from build123d import *

# Parameters (mm, degrees)
EXTRUDE_THIN1_DEPTH = 44
SKETCH2_R           = 2.58
CUT_EXTRUDE1_DEPTH  = 10
FILLET1_R           = 18
FILLET2_R           = 18
FILLET3_R           = 18
FILLET4_R           = 18
FILLET5_R           = 1
FILLET6_R           = 1
SKETCH11_R          = 5
SKETCH11_R_2        = 0.6
CUT_EXTRUDE2_DEPTH  = 10
SKETCH12_R          = 5
SKETCH12_R_2        = 0.6
CUT_EXTRUDE3_DEPTH  = 10


with BuildPart() as part:
    # Sketch1 → Extrude-Thin1 (new body)
    with BuildSketch(Plane(origin=(0, 0, 0), x_dir=(1, 0, 0), z_dir=(0, 1, 0))):
        Polygon((31, 57), (31, 0), (-31, 0), (-31, 57), (-32, 57), (-32, -1), (32, -1), (32, 57), align=None)
    extrude(amount=EXTRUDE_THIN1_DEPTH)

    # Sketch2 → Cut-Extrude1 (cut)
    with BuildSketch(Plane(origin=(32, 0, 0), x_dir=(0, 0, -1), z_dir=(1, 0, 0))):
        with Locations((39, 22)):
            Circle(SKETCH2_R)
    extrude(amount=-CUT_EXTRUDE1_DEPTH, mode=Mode.SUBTRACT)

    # Fillet1
    fillet1_edges = [part.edges().sort_by_distance(p)[0] for p in [
        (31.5, 0, -57),
    ]]
    fillet(fillet1_edges, radius=FILLET1_R)

    # Fillet2
    fillet2_edges = [part.edges().sort_by_distance(p)[0] for p in [
        (31.5, 44, -57),
    ]]
    fillet(fillet2_edges, radius=FILLET2_R)

    # Fillet3
    fillet3_edges = [part.edges().sort_by_distance(p)[0] for p in [
        (-31.5, 44, -57),
    ]]
    fillet(fillet3_edges, radius=FILLET3_R)

    # Fillet4
    fillet4_edges = [part.edges().sort_by_distance(p)[0] for p in [
        (-31.5, 0, -57),
    ]]
    fillet(fillet4_edges, radius=FILLET4_R)

    # Fillet5
    fillet5_edges = [part.edges().sort_by_distance(p)[0] for p in [
        (-32, 22, 1),
    ]]
    fillet(fillet5_edges, radius=FILLET5_R)

    # Fillet6
    fillet6_edges = [part.edges().sort_by_distance(p)[0] for p in [
        (32, 22, 1),
    ]]
    fillet(fillet6_edges, radius=FILLET6_R)

    # Sketch11 → Cut-Extrude2 (cut)
    with BuildSketch(Plane.ZY.offset(32)):
        with Locations((-38.961003009, 22)):
            Circle(SKETCH11_R)
        with Locations((-38.961003009, 30)):
            Circle(SKETCH11_R_2)
        with Locations((-30.961003009, 22)):
            Circle(SKETCH11_R_2)
        with Locations((-38.961003009, 14)):
            Circle(SKETCH11_R_2)
        with Locations((-46.961003009, 22)):
            Circle(SKETCH11_R_2)
        with Locations((-44.617857259, 27.656854249)):
            Circle(SKETCH11_R_2)
        with Locations((-33.30414876, 27.656854249)):
            Circle(SKETCH11_R_2)
        with Locations((-33.30414876, 16.343145751)):
            Circle(SKETCH11_R_2)
        with Locations((-44.617857259, 16.343145751)):
            Circle(SKETCH11_R_2)
    extrude(amount=-CUT_EXTRUDE2_DEPTH, mode=Mode.SUBTRACT)

    # Sketch12 → Cut-Extrude3 (cut)
    with BuildSketch(Plane.XY.offset(1)):
        with Locations((0, 22)):
            Circle(SKETCH12_R)
        with Locations((0, 30)):
            Circle(SKETCH12_R_2)
        with Locations((5.656854249, 27.656854249)):
            Circle(SKETCH12_R_2)
        with Locations((8, 22)):
            Circle(SKETCH12_R_2)
        with Locations((5.656854249, 16.343145751)):
            Circle(SKETCH12_R_2)
        with Locations((0, 14)):
            Circle(SKETCH12_R_2)
        with Locations((-5.656854249, 16.343145751)):
            Circle(SKETCH12_R_2)
        with Locations((-8, 22)):
            Circle(SKETCH12_R_2)
        with Locations((-5.656854249, 27.656854249)):
            Circle(SKETCH12_R_2)
    extrude(amount=-CUT_EXTRUDE3_DEPTH, mode=Mode.SUBTRACT)


solid = part.part
Build history of the part. All positions in model axes, mm. A direction names the side the tool comes from. Round coordinates to 2 decimals unless told otherwise and drop trailing zeros. Write each loop counter-clockwise with the first axis right and the second up, starting at its lowest first coordinate (ties: lowest second). Pieces come first, ordered by that corner, then holes. Notation, with made-up numbers: M 33.25,-5 L 56.25,-5 A7 cw 56.25,5 Z; hole C -9.75,-7 d2. An arc over 180 degrees is marked long. Answer as a JSON object with one key per item and string values. Group by question number.
(1) Cut at C-C (y = 41). Give the cut face in (x, z), and give its area (3 significant figures).
(2) Flat gauge pins, fed straight in: pin 1 (16 mm diameter, centred on x = 0, y = 22, fed in from -Z); pin 2 (0.7 mm diameter, centred on y = 22, z = -30.96, fed in from -X). Where does each tip first touch, or does it go through?
(3) Cut at D-D (x = -21). Give the cut face in (y, z).
(4) Cut at B-B (x = -2.5). Give the cut face in (y, z), and give its area (3 significant figures).
(5) Mould opens along X. For faces 1 (the flat face through (32, 22, -28)), 2 (the cylindrical face through (-1.08, 17.12, 0.51)), 3 (the cylindrical face through (-31.507, 17.564, -36.654)) say: pulls with the +X half, pulls with the -X half, needs draft (parallel to the pull), parting line crosses it, or undercut.
(6) Which spindle directions (+Z, -Z, +X, -X, +Y, -Y) get a long thin tool onto all of the face, cutting with end or side? Do faces 4 (the flat face through (31, 22, -29)), 5 (the flat face through (-0.4, 16.8, 1)). Say none if no direction does.
(7) Drill centre lines: L1, parallel to X at y = 35.5, z = -34.5; L2, parallel to Z at x = 19.5, y = 3.5. Where is each one in solid material? Low to high.
(8) Cut at A-A (z = -7). Give the cut face in (x, y), and give its area (3 significant figures).
Responses:
{
 "1": {"outline": "M -32,-48.95 L -31,-48.95 L -31,0 L 31,0 L 31,-48.95 L 32,-48.95 L 32,0 A1 ccw 31,1 L -31,1 A1 ccw -32,0 Z", "area": "161 mm2"},
 "2": {"pin 1": "stops at z = 0", "pin 2": "stops at x = 31"},
 "3": {"outline": "M 0,0 L 44,0 L 44,1 L 0,1 Z"},
 "4": {"outline": "M 0,0 L 17.67,0 L 17.67,1 L 0,1 Z; M 26.33,0 L 44,0 L 44,1 L 26.33,1 Z", "area": "35.3 mm2"},
 "5": {"face 1": "pulls with the +X half", "face 2": "undercut", "face 3": "needs draft"},
 "6": {"face 4": "-Z, +Y, -Y", "face 5": "+Z, +X, -X, +Y, -Y"},
 "7": {"L1": "x = -32 to -31, 31 to 32", "L2": "z = 0 to 1"},
 "8": {"outline": "M -32,0 L -31,0 L -31,44 L -32,44 Z; M 31,0 L 32,0 L 32,44 L 31,44 Z", "area": "88.0 mm2"}
}
